Check sheet for the drawn part. Datum: minimum x, y, z corner. Units: mm. A direction names the side the tool comes from. Give positions to 0.01 mm unless a question says otherwise; leave off trailing zeros. Write each loop counter-clockwise with the first axis right and the second up, starting at its lowest first coordinate (ties: lowest second). Pieces come first, ordered by that corner, then holes. Notation, with made-up numbers: (86.25, -29) -> (95.25, -29) arc R24 cw to (95.25, -9) -> close; hole circle Ø9 at (-39, 89). An arc over 180 degrees is marked (long way). Write item = value, one per line. Start each with the question number.
1. Cross-section at C-C, the plane z = 7.5. Record the cut outline in (x, y).
2. Cross-section at D-D, the plane x = 25.5. Record the cut outline in (y, z).
3. Depth check by flat-ended pin: P1, Ø10, axis at y = 5, z = 32, coming from the +X side; P2, Ø1.5, axis at x = 30, y = 15.5, coming from the +Z side; P3, Ø1, axis at x = 6.5, z = 31, coming from the -Y side; P4, Ø12.5, axis at x = 29.5, y = 34.5, coming from the -Z side. Enter the tip coordinate at first touch or a pass-through.
4. Cross-section at A-A, the plane z = 32. Record the cut outline in (x, y), plus the area to 3 significant figures.
5. Set-up check for the marked faces 1, 2 and 3: record each of +Z, -Z, +X, -X, +Y, -Y from which the full face is reachable in a straight line by a thin tool's end or side.
6. Cross-section at B-B, the plane x = 32. Record the cut outline in (y, z).
7. Thickness scan on line 1 along X through (y, z) = (3.5, 32); line 2 along X through (y, z) = (3.15, 7.5); line 3 along X through (y, z) = (1, 7). Record the ranges inside material, lowest first.
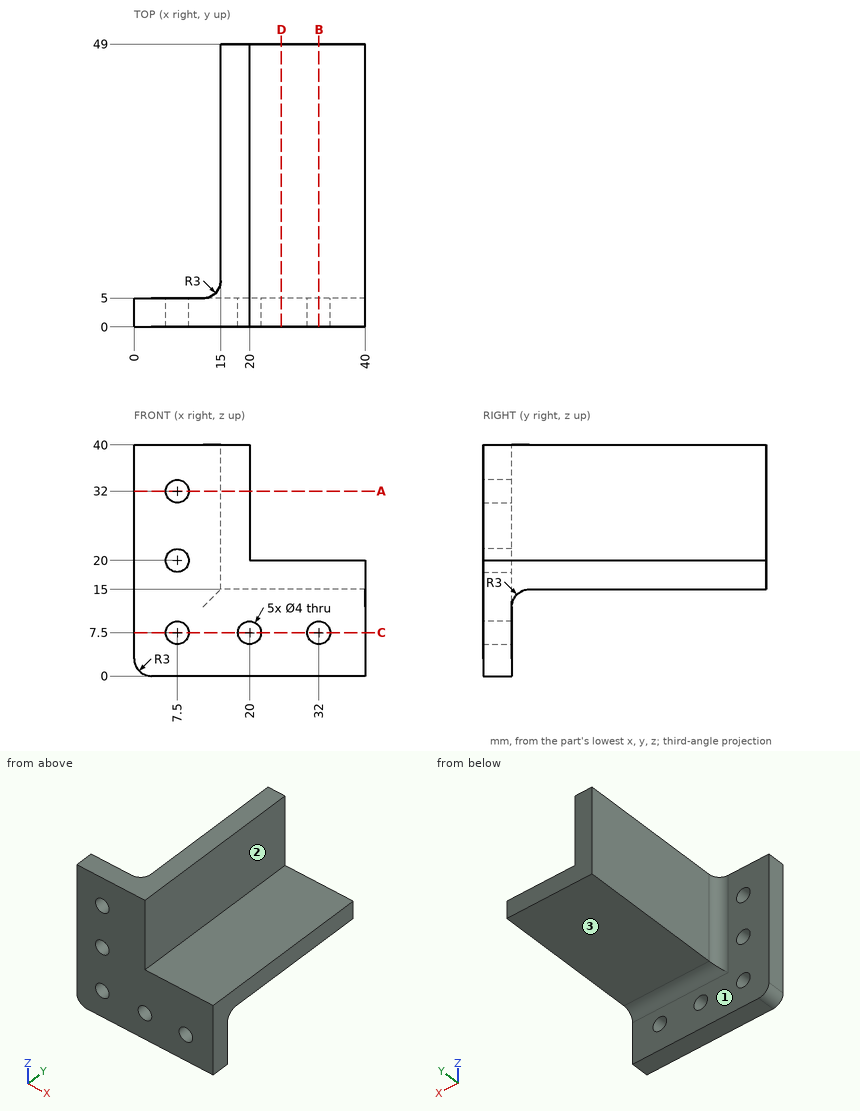
Answers:
q1.outline = (0, 0) -> (5.5, 0) -> (5.5, 5) -> (0, 5) -> close; (9.5, 0) -> (18, 0) -> (18, 5) -> (9.5, 5) -> close; (22, 0) -> (30, 0) -> (30, 5) -> (22, 5) -> close; (34, 0) -> (40, 0) -> (40, 5) -> (34, 5) -> close
q2.outline = (0, 0) -> (5, 0) -> (5, 12) arc R3 cw to (8, 15) -> (49, 15) -> (49, 20) -> (0, 20) -> close
q3.P1 = 20
q3.P2 = 20
q3.P3 = through
q3.P4 = 15
q4.outline = (0, 0) -> (5.5, 0) -> (5.5, 5) -> (0, 5) -> close; (9.5, 0) -> (20, 0) -> (20, 49) -> (15, 49) -> (15, 8) arc R3 cw to (12, 5) -> (9.5, 5) -> close
q4.area = 302 mm^2
q5.face_1 = -Z, -X, +Y
q5.face_2 = +Z, +X, +Y, -Y
q5.face_3 = -Z, +X, -X, +Y
q6.outline = (0, 0) -> (5, 0) -> (5, 5.5) -> (0, 5.5) -> close; (0, 9.5) -> (5, 9.5) -> (5, 12) arc R3 cw to (8, 15) -> (49, 15) -> (49, 20) -> (0, 20) -> close
q7.line_1 = 0 to 5.5, 9.5 to 20
q7.line_2 = 0 to 5.5, 9.5 to 18, 22 to 30, 34 to 40
q7.line_3 = 0 to 5.56, 9.44 to 18.06, 21.94 to 30.06, 33.94 to 40
